```python
from build123d import *

# Parameters (mm, degrees)
EXTRUDE_1_DEPTH     = 25
SKETCH_2_R          = 19.5
EXTRUDE_2_DEPTH     = 73
SKETCH_3_R          = 7.5
EXTRUDE_3_DEPTH     = 2
EXTRUDE_4_DEPTH     = 454
SKETCH_5_R          = 10
CUT_EXTRUDE_1_DEPTH = 410
EXTRUDE_5_DEPTH     = 19
SKETCH_7_R          = 3.25
CUT_EXTRUDE_2_DEPTH = 19


with BuildPart() as part:
    # 草图1 → 凸台-拉伸1 (new body)
    with BuildSketch(Plane.XY):
        with BuildLine():
            Line((-20, 0), (-20, 44.928932188))
            ThreePointArc((-20, 44.928932188), (-19.619397663, 46.84234935), (-18.535533906, 48.464466094))
            Line((-18.535533906, 48.464466094), (-13.464466094, 53.535533906))
            ThreePointArc((-13.464466094, 53.535533906), (-11.84234935, 54.619397663), (-9.928932188, 55))
            Line((-9.928932188, 55), (9.928932188, 55))
            ThreePointArc((9.928932188, 55), (11.84234935, 54.619397663), (13.464466094, 53.535533906))
            Line((13.464466094, 53.535533906), (18.535533906, 48.464466094))
            ThreePointArc((18.535533906, 48.464466094), (19.619397663, 46.84234935), (20, 44.928932188))
            Line((20, 44.928932188), (20, 0))
            ThreePointArc((20, 0), (0, -20), (-20, 0))
        make_face()
    extrude(amount=EXTRUDE_1_DEPTH)

    # 草图2 → 凸台-拉伸2 (add)
    with BuildSketch(Plane.XY.offset(25)):
        Circle(SKETCH_2_R)
    extrude(amount=EXTRUDE_2_DEPTH)

    # 草图3 → 凸台-拉伸3 (add)
    with BuildSketch(Plane.XY.offset(98)):
        Circle(SKETCH_3_R)
    extrude(amount=EXTRUDE_3_DEPTH)

    # 草图4 → 凸台-拉伸4 (add)
    with BuildSketch(Plane.XY.offset(25)):
        with BuildLine():
            Line((-11.576521962, 54), (-13.87569737, 36.861457087))
            ThreePointArc((-13.87569737, 36.861457087), (0, 21), (13.87569737, 36.861457087))
            Line((13.87569737, 36.861457087), (11.576521962, 54))
            Line((11.576521962, 54), (-11.576521962, 54))
        make_face()
    extrude(amount=EXTRUDE_4_DEPTH)

    # 草图5 → 切除-拉伸1 (cut)
    with BuildSketch(Plane.XY.offset(479)):
        with Locations((0, 35)):
            Circle(SKETCH_5_R)
    extrude(amount=-CUT_EXTRUDE_1_DEPTH, mode=Mode.SUBTRACT)

    # 草图6 → 凸台-拉伸5 (add)
    with BuildSketch(Plane(origin=(0, 0, 0), x_dir=(-1, 0, 0), z_dir=(0, 0, -1))):
        with BuildLine():
            Line((-4.358898944, 44), (4.358898944, 44))
            ThreePointArc((4.358898944, 44), (7.071067812, 42.071067812), (9, 39.358898944))
            Line((9, 39.358898944), (9, 30.641101056))
            ThreePointArc((9, 30.641101056), (7.071067812, 27.928932188), (4.358898944, 26))
            Line((4.358898944, 26), (-4.358898944, 26))
            ThreePointArc((-4.358898944, 26), (-7.071067812, 27.928932188), (-9, 30.641101056))
            Line((-9, 30.641101056), (-9, 39.358898944))
            ThreePointArc((-9, 39.358898944), (-7.071067812, 42.071067812), (-4.358898944, 44))
        make_face()
    extrude(amount=EXTRUDE_5_DEPTH)

    # 草图7 → 切除-拉伸2 (cut)
    with BuildSketch(Plane(origin=(9, 0, 0), x_dir=(0, 0, -1), z_dir=(1, 0, 0))):
        with Locations((12, 35)):
            Circle(SKETCH_7_R)
    extrude(amount=-CUT_EXTRUDE_2_DEPTH, mode=Mode.SUBTRACT)


solid = part.part
```
Geometry: final body of the model. Coordinates: model frame, mm. A direction names the side the tool comes from. Round coordinates to 2 decimals unless told otherwise and drop trailing zeros. Order: outer loops, then holes, each group sorted by start corner. A loop starts at its lowest first (then second) coordinate and runs counter-clockwise, first axis right, second up. Notation, with made-up numbers: (-31, 26.5) -> (9, 26.5) arc R21 cw to (9, 65.5) -> close; hole circle Ø11 at (17, -3). An arc over 180 degrees is marked (long way). Use CSV: the item, a comma, the result in double quotes. Start each with the question number.
1) Section D-D (y = -15). Return the cut outline in (x, z).
2) Section B-B (z = 284.5). Return the cut outline in (x, y).
3) Set-up query: faces 1 (the face through (9, 35, -7)), 2 (the face through (0, 54, 249)), 3 (the face through (0, 44, -9)), 4 (the face through (-2.17, 25.24, 276.87)). Return all of +Z, -Z, +X, -X, +Y, -Y with unobstructed straight access to the full face (end or side cutting, diameter ignored); none if empty.
4) Section C-C (z = 15). Return the cut outline in (x, y).
5) First-contact query: pin 1 Ø19.5 at (x, y) = (-3, 6) entering from +Z; pin 2 Ø9.5 at (y, z) = (34.5, -11) entering from -X; pin 3 Ø3 at (x, y) = (4, 14) entering from -Z; pin 4 Ø4 at (y, z) = (35, -12) entering from +X. Flat tips, straight axial feed; report the tip coordinate or a pass-through.
6) Draft query along Y for faces 5 (the face through (8, 0, 98)), 6 (the face through (-12.71, 45.55, 248.82)), 7 (the face through (0, 26, -9)), 8 (the face through (20, 23, 12)). Return one class per face: +Y half, -Y half, draft (parallel to the pull), parting line (faces both ways), or undercut.
7) Section A-A (x = 0). Return the cut outline in (y, z), and give its area (3 significant figures).
8) Material intervals for line 1 along Y through (x, z) = (-1, -12); line 2 along Y through (x, z) = (1, 49.5); line 3 along Y through (x, z) = (6, 92), sorted ascending. Write a range as from..to.
Returned:
1,outline,"(-13.23, 0) -> (13.23, 0) -> (13.23, 25) -> (12.46, 25) -> (12.46, 98) -> (-12.46, 98) -> (-12.46, 25) -> (-13.23, 25) -> close"
2,outline,"(-13.88, 36.86) arc R14 ccw (long way) to (13.88, 36.86) -> (11.58, 54) -> (-11.58, 54) -> close; hole circle Ø20 at (0, 35)"
3,face 1,"-Z, +X, +Y, -Y"
3,face 2,"+Z, +X, -X, +Y"
3,face 3,"-Z, +X, -X, +Y"
3,face 4,"+Z"
4,outline,"(-20, 0) arc R20 ccw to (20, 0) -> (20, 44.93) arc R5 ccw to (18.54, 48.46) -> (13.46, 53.54) arc R5 ccw to (9.93, 55) -> (-9.93, 55) arc R5 ccw to (-13.46, 53.54) -> (-18.54, 48.46) arc R5 ccw to (-20, 44.93) -> close"
5,pin 1,"stops at z = 100"
5,pin 2,"stops at x = -9"
5,pin 3,"stops at z = 0"
5,pin 4,"passes through"
6,face 5,"undercut"
6,face 6,"+Y half"
6,face 7,"-Y half"
6,face 8,"draft"
7,outline,"(-20, 0) -> (26, 0) -> (26, -19) -> (44, -19) -> (44, 0) -> (55, 0) -> (55, 25) -> (54, 25) -> (54, 479) -> (45, 479) -> (45, 69) -> (25, 69) -> (25, 479) -> (21, 479) -> (21, 25) -> (19.5, 25) -> (19.5, 98) -> (7.5, 98) -> (7.5, 100) -> (-7.5, 100) -> (-7.5, 98) -> (-19.5, 98) -> (-19.5, 25) -> (-20, 25) -> close; hole circle Ø6.5 at (35, -12)"
7,area,"11,800 mm²"
8,line 1,"y = 26..31.75, 38.25..44"
8,line 2,"y = -19.47..19.47, 21.04..54"
8,line 3,"y = -18.55..18.55, 22.35..27, 43..54"
